Autodesk Inventor part; units mm, degrees
ref_plane "YZ Plane" through (0, 0, 0) normal (1, 0, 0) x (0, 1, 0)
ref_plane "XZ Plane" through (0, 0, 0) normal (0, 1, 0) x (-1, 0, 0)
ref_plane "XY Plane" through (0, 0, 0) normal (0, 0, 1) x (1, 0, 0)
sketch "Sketch1" plane through (0, 0, 0) normal (0, 0, 1) x (1, 0, 0)
  line L0 (0, 0) -> (30, 0)
  line L1 (30, 0) -> (30, 4)
  line L2 (30, 4) -> (0, 4)
  line L3 (0, 4) -> (0, 0)
  line L4 (15, 4) -> (11, 4)
  line L5 (15, 4) -> (19, 4)
  line L6 (11, 4) -> (11, 60)
  line L7 (19, 4) -> (19, 60)
  line L8 (11, 60) -> (19, 60)
  circle A0 centre (15, 60) radius 7.5
  circle A1 centre (15, 60) radius 12.5
  arc A2 (11, 48.1573) -> (19, 48.1573) centre (15, 60) ccw
  arc A3 (11, 53.6557) -> (19, 53.6557) centre (15, 60) ccw
  dimension "d0" = 30
  dimension "d1" = 4
  dimension "d2" = 4
  dimension "d3" = 4
  dimension "d5" = 60
  dimension "d6" = 15
  dimension "d7" = 25
extrude "Extrusion1" add sketch "Sketch1" along normal mid plane 12 contours L3 L2 L1 L0 | L6 A1 L7 L2
extrude "Extrusion2" add sketch "Sketch1" along normal mid plane 20 contours A1 L7 A0 L6 | L6 A0 L7 A1
sketch "Sketch2" plane through (19, 4, 6) normal (0, 1, 0) x (1, 0, 0)
  line L0 (0, 12) -> (0, 0)
  line L1 (11, 0) -> (0, 0)
  line L2 (11, 12) -> (11, 0)
  line L3 (0, 12) -> (11, 12)
  line L4 (0, 6) -> (11, 6)
  point P0 (-19, 6)
  point P1 (5.5, 6)
hole "Hole1" at (24.5, 4, 0) direction (0, -1, 0) diameter 3.5 end up to surface
ref_plane "Work Plane1" through (15, 4, -6) normal (-1, 0, 0) x (0, 0, 1)
mirror "Mirror1" about plane through (15, 4, -6) normal (-1, 0, 0) of "Hole1"
sketch "Sketch3" plane through (15, 60, 10) normal (0, 0, 1) x (1, 0, 0)
  circle A0 centre (0, 0) radius 7.5
  line L0 (0, 0) -> (2.5652, -7.0477)
  line L1 (0, 0) -> (-2.5652, -7.0477)
  line L2 (0, -74.5) -> (0, 27)
  line L3 (0, -7.5) -> (0, -2.25)
  line L4 (0, 0) -> (-7.5, 0)
  line L5 (7.5, 0) -> (0, 0)
  line L6 (3.75, 0) -> (4.5689, -2.25)
  line L7 (0, -3.75) -> (4.5689, -3.75)
  line L8 (4.5689, -3.75) -> (4.5689, -2.25)
  line L9 (2.9311, -2.25) -> (0, -2.25)
  line L10 (0, -2.25) -> (0, -3.75)
  line L11 (3.75, 0) -> (2.9311, -2.25)
  arc A1 (-2.5652, -7.0477) -> (2.5652, -7.0477) centre (0, 0) ccw
  point P0 (-15, -60)
  point P1 (-3.75, 0)
  dimension "d19" = 20
  dimension "d20" = 20
  dimension "d21" = 70
  dimension "d22" = 1.5
  dimension "d23" = 70
  dimension "d24" = 4.5689
  dimension "d25" = 2.9311
extrude "Extrusion3" add sketch "Sketch3" against normal up to surface (20 mm away) contours L1 L2 A0 | L0 L9 L2 | L2 L7 L0 A0 | L9 L11 L6 L8 L7 L0 | L0 L7 L2 L9
mirror "Mirror2" about plane through (15, 4, -6) normal (-1, 0, 0) of "Extrusion3"
equation "\"d2\" = d3"
equation "\"d20\" = d19"
equation "\"d23\" = d21"
properties part number "frontSight"
Could you check a few things on this model? Use its own coordinates, in mm. A direction names the side the tool comes from. Round coordinates to 2 decimals unless told otherwise and drop trailing zeros. Write each loop counter-clockwise with the first axis right and the second up, starting at its lowest first coordinate (ties: lowest second). Pieces come first, ordered by that corner, then holes. Notation, with made-up numbers: (53, -1.75) - (80, -1.75) arc R23 cw to (80, 11.25) - close; hole circle Ø5 at (30.25, 75.25). An arc over 180 degrees is marked (long way). Put each result on its own line as item: value. Start each with the question number.
(1) Will these pins go through, and if not, where does the flat tip stop? pin 1 (5 mm diameter, centred on x = 9.5, y = 40, fed in from -Z); pin 2 (1.2 mm diameter, centred on y = 56.5, z = 3, fed in from +X); pin 3 (5.5 mm diameter, centred on x = 27, z = 1.5, fed in from +Y).
(2) I want a section at D-D, the plane z = -5. Please give me the cut outline in (x, y), plus the area to 3 significant figures.
(3) I want a section at A-A, the plane x = 20.25. Please give me the cut outline in (y, z), plus the area to 3 significant figures.
(4) I want a section at B-B, the plane z = -0.5. Give the number of separate pieces and of enclosed holes in the cut face, plus the area to 3 significant figures.
(5) I need wall thicknesses on probe 1 along X at (y, z) = (0.9, 0); probe 2 along Z at (x, y) = (5.5, 3.15); probe 3 along Y at (x, z) = (24, -4.5). Which ranges of each line are inside material? Lowest first, please.
(6) For faces 1 (the flat face through (0, 2, 0)), 2 (the flat face through (25.8, 4, -1.4)), 3 (the flat face through (11, 26, 0)), 4 (the flat face through (15.4, 58.9, 0.1)), which set-ups out of +Z, -Z, +X, -X, +Y, -Y let a thin tool reach every point of the face, with its end or its side?
(7) I want a section at C-C, the plane y = 25. Please give me the cut outline in (x, z).
(8) Thinking about a two-plate mould opening in Y: for faces 5 (the flat face through (6.8, 4, -1.4)), 6 (the cylindrical face through (15.1, 47.5, 8)), 7 (the cylindrical face through (7.21, 1.97, -0.38)), which applies, released by +Y, released by -Y, zero draft, split by the parting line, or undercut?
Here are the results:
1. pin 1: stops at z = -6
1. pin 2: stops at x = 27.16
1. pin 3: stops at y = 68.41
2. outline: (0, 0) - (30, 0) - (30, 4) - (19, 4) - (19, 48.16) arc R12.5 ccw (long way) to (11, 48.16) - (11, 4) - (0, 4) - close; hole (10.43, 56.25) - (10.43, 57.75) - (11.25, 60) - (12.07, 57.75) - (14.18, 57.75) - (15, 60) - (15.82, 57.75) - (17.93, 57.75) - (18.75, 60) - (19.57, 57.75) - (19.57, 56.25) - (16.36, 56.25) - (17.57, 52.95) arc R7.5 ccw (long way) to (11, 53.66) arc R7.5 ccw to (12.43, 52.95) - (13.64, 56.25) - close
2. area: 818 mm^2
3. outline: (0, -6) - (4, -6) - (4, 6) - (0, 6) - close; (48.66, -10) - (54.64, -10) - (54.64, 10) - (48.66, 10) - close; (65.36, -10) - (71.34, -10) - (71.34, 10) - (65.36, 10) - close
3. area: 288 mm^2
4. separate pieces: 3
4. enclosed holes: 1
4. area: 791 mm^2
5. probe 1: x = 0 to 3.75, 7.25 to 22.75, 26.25 to 30
5. probe 2: z = -6 to -1.75, 1.75 to 6
5. probe 3: y = 0 to 4, 51.33 to 68.67
6. face 1: +Z, -Z, -X, +Y, -Y
6. face 2: +Z, -Z, +X
6. face 3: +Z, -Z, -X
6. face 4: +Z, -Z
7. outline: (11, -6) - (19, -6) - (19, 6) - (11, 6) - close
8. face 5: undercut
8. face 6: released by -Y
8. face 7: zero draft
